For this review, take the finished solid that the model builds, in its own axes (mm). Face numbers are marked on the shaded views. Give positions to 0.01 mm unless a question says otherwise; leave off trailing zeros. Write each loop counter-clockwise with the first axis right and the second up, starting at its lowest first coordinate (ties: lowest second). Pieces come first, ordered by that corner, then holes. Notation, with made-up numbers: M 43.5,77 L 99.5,77 A18 cw 99.5,106 Z; hole C -19.75,2.5 d10. An arc over 180 degrees is marked long. Write item = value, one per line.
```python
from build123d import *

# Parameters (mm, degrees)
SKETCH1_R                = 90
BOSS_EXTRUDE1_DEPTH      = 5
SKETCH2_W                = 15
SKETCH2_H                = 35
BOSS_EXTRUDE2_DEPTH      = 110
CUT_EXTRUDE1_DEPTH       = 36
SKETCH4_R                = 2.18255
CUT_EXTRUDE2_DEPTH       = 62
BOSS_EXTRUDE4_DEPTH      = 15
BOSS_EXTRUDE4_DEPTH_BACK = 30
SKETCH6_W                = 30.491916349
SKETCH6_H                = 4.74874107
SKETCH6_H_2              = 4.248873589


with BuildPart() as part:
    # Sketch1 → Boss-Extrude1 (new body)
    with BuildSketch(Plane(origin=(0, 0, 0), x_dir=(1, 0, 0), z_dir=(0, 1, 0))):
        with Locations(Location((0, 0, 0), (0, 0, 270))):
            Circle(SKETCH1_R)
    extrude(amount=BOSS_EXTRUDE1_DEPTH)

    # Sketch2 → Boss-Extrude2 (add)
    with BuildSketch(Plane(origin=(0, 5, 0), x_dir=(1, 0, 0), z_dir=(0, 1, 0))):
        Rectangle(SKETCH2_W, SKETCH2_H)
    extrude(amount=BOSS_EXTRUDE2_DEPTH)

    # Sketch3 → Cut-Extrude1 (cut)
    with BuildSketch(Plane.XY.offset(17.5)):
        Polygon((-2.373551685, 115), (2.826448315, 115), (5.726448315, 109.977052658), (-5.273551685, 109.977052658), align=None)
    extrude(amount=-CUT_EXTRUDE1_DEPTH, mode=Mode.SUBTRACT)

    # Sketch4 → Cut-Extrude2 (cut)
    with BuildSketch(Plane(origin=(0, 0, 0), x_dir=(-1, 0, 0), z_dir=(0, -1, 0))):
        with Locations(Location((-26.585, 79.907325251, 0), (0, 0, 90))):
            Circle(SKETCH4_R)
        with Locations(Location((26.585, 79.907325251, 0), (0, 0, 90))):
            Circle(SKETCH4_R)
        with Locations(Location((82.310329065, -16.825152102, 0), (0, 0, 90))):
            Circle(SKETCH4_R)
        with Locations(Location((56.093218167, -63.082173149, 0), (0, 0, 90))):
            Circle(SKETCH4_R)
        with Locations(Location((26.585, -79.907325251, 0), (0, 0, 90))):
            Circle(SKETCH4_R)
        with Locations(Location((-26.585, -79.907325251, 0), (0, 0, 90))):
            Circle(SKETCH4_R)
        with Locations(Location((-53.346563788, -64.612502947, 0), (0, 0, 90))):
            Circle(SKETCH4_R)
        with Locations(Location((-82.245302282, -19.978089739, 0), (0, 0, 90))):
            Circle(SKETCH4_R)
    extrude(amount=-CUT_EXTRUDE2_DEPTH, mode=Mode.SUBTRACT)

    # Sketch6 → Boss-Extrude4 (add, two sides: drawn at the far end of the back side and taken through both)
    with BuildSketch(Plane(origin=(7.5, 0, 0), x_dir=(0, 0, -1), z_dir=(1, 0, 0)).offset(-BOSS_EXTRUDE4_DEPTH_BACK)):
        with Locations((0.124966871, 55.070581362)):
            Rectangle(SKETCH6_W, SKETCH6_H)
        with Locations((0.124966871, 41.699126242)):
            Rectangle(SKETCH6_W, SKETCH6_H_2)
    extrude(amount=BOSS_EXTRUDE4_DEPTH + BOSS_EXTRUDE4_DEPTH_BACK)


solid = part.part
```
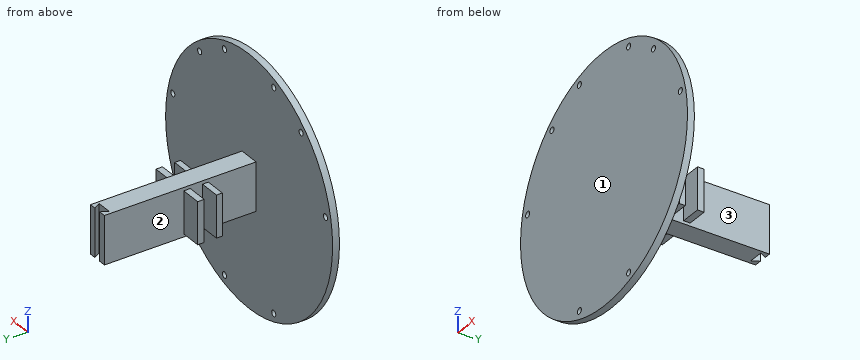
1. We need section B-B, the plane z = 0. Write out the cut boundary in (x, y).
Responses:
outline = M -90,0 L 90,0 L 90,5 L 7.5,5 L 7.5,39.57 L 22.5,39.57 L 22.5,43.82 L 7.5,43.82 L 7.5,52.7 L 22.5,52.7 L 22.5,57.44 L 7.5,57.44 L 7.5,115 L 2.83,115 L 5.73,109.98 L -5.27,109.98 L -2.37,115 L -7.5,115 L -7.5,57.44 L -22.5,57.44 L -22.5,52.7 L -7.5,52.7 L -7.5,43.82 L -22.5,43.82 L -22.5,39.57 L -7.5,39.57 L -7.5,5 L -90,5 Z
2. We need section D-D, the plane z = 74.5. Write out the cut boundary in (x, y).
Responses:
outline = M -50.5,0 L 50.5,0 L 50.5,5 L -50.5,5 Z
3. We need section A-A, the plane x = 0. Write out the cut boundary in (y, z), then the cut area to 3 significant figures.
Responses:
outline = M 0,-90 L 5,-90 L 5,-17.5 L 109.98,-17.5 L 109.98,17.5 L 5,17.5 L 5,90 L 0,90 Z
area = 4,570 mm2
4. The part is to be moulded in two halves that separate along Y. For the marked faces 1, 2 and 3, say which applies: +Y half, -Y half, draft (parallel to the pull), parting line (faces both ways), or undercut.
Responses:
face_1 = -Y half
face_2 = undercut
face_3 = undercut
5. We need section C-C, the plane y = 29. Write out the cut boundary in (x, z).
Responses:
outline = M -7.5,-17.5 L 7.5,-17.5 L 7.5,17.5 L -7.5,17.5 Z
6. For line 1 along Y through (x, z) = (3, 40.5); line 2 along X through (y, z) = (35.5, 5), list the stretches that pass through material, from the lowest coordinate up. Write a range as from..to.
Responses:
line_1 = 0..5
line_2 = -7.5..7.5
7. Insertion check: P1, Ø2.5, axis at x = 82.25, z = 19.98, coming from the -Y side (1 decimal); P2, Ø7.5, axis at x = -1.5, y = 51.5, coming from the +Z side; P3, Ø3.5, axis at y = 42, z = -2, coming from the -X side; P4, Ø5, axis at x = 53.35, z = 64.61, coming from the +Y side. Each pin has a flat end and moves straight along its axis. Give the tip position at first contact, or say it passes through.
Responses:
P1 = through
P2 = 17.5
P3 = -22.5
P4 = 5
